Work out the finished part from the listing and answer in its coordinate system (mm). A direction names the side the tool comes from. Round coordinates to 2 decimals unless told otherwise and drop trailing zeros. Order: outer loops, then holes, each group sorted by start corner. A loop starts at its lowest first (then second) coordinate and runs counter-clockwise, first axis right, second up. Notation, with made-up numbers: M 21.25,-19 L 58.25,-19 A17 cw 58.25,-5 Z; hole C 33,-19 d2. An arc over 180 degrees is marked long. Return JSON: item names as keys, results as strings.
from build123d import *

# Parameters (mm, degrees)
BOX005_W                             = 145
BOX005_H                             = 15
BOX005_DEPTH                         = 182.3
BOX006_W                             = 19
BOX006_H                             = 163
BOX006_DEPTH                         = 13
BOX007_W                             = 112
BOX007_H                             = 172
BOX007_DEPTH                         = 1.5
BOX008_W                             = 11
BOX008_H                             = 32
BOX008_DEPTH                         = 2
BOX009_W                             = 3
BOX009_H                             = 24
BOX009_DEPTH                         = 17
BOX010_W                             = 60
BOX010_H                             = 32
BOX010_DEPTH                         = 5
BOX011_W                             = 15
BOX011_H                             = 80
BOX011_DEPTH                         = 5
BOX012_W                             = 5
BOX012_H                             = 70
BOX012_DEPTH                         = 3
LINEARPATTERN001_COUNT               = 2
LINEARPATTERN001_PITCH               = 80
FILLET_R                             = 1
FILLET001_R                          = 1
CYLINDER002_R                        = 1
CYLINDER002_DEPTH                    = 20
CYLINDER002_LINEARPATTERN002_2_R     = 1
CYLINDER002_LINEARPATTERN002_2_DEPTH = 20
LINEARPATTERN003_COUNT               = 2
LINEARPATTERN003_PITCH               = 170
BOX013_W                             = 11
BOX013_H                             = 165
BOX013_DEPTH                         = 4
CYLINDER004_R                        = 1
CYLINDER004_DEPTH                    = 3
CYLINDER004_LINEARPATTERN006_2_R     = 1
CYLINDER004_LINEARPATTERN006_2_DEPTH = 3
LINEARPATTERN007_COUNT               = 8
LINEARPATTERN007_PITCH               = 20
CYLINDER005_R                        = 3
CYLINDER005_DEPTH                    = 10
CYLINDER005_LINEARPATTERN008_2_R     = 3
CYLINDER005_LINEARPATTERN008_2_DEPTH = 10
LINEARPATTERN009_COUNT               = 2
LINEARPATTERN009_PITCH               = 170


with BuildPart() as part:
    # Box005 → Box005 (join)
    with BuildSketch(Plane(origin=(0, 182, -11), x_dir=(1, 0, 0), z_dir=(0, -1, 0))):
        with Locations((72.5, 7.5)):
            Rectangle(BOX005_W, BOX005_H)
    extrude(amount=BOX005_DEPTH)

    # Box006 → Box006 (cut)
    with BuildSketch(Plane(origin=(2, 8, -9), x_dir=(1, 0, 0), z_dir=(0, 0, 1))):
        with Locations((9.5, 81.5)):
            Rectangle(BOX006_W, BOX006_H)
    extrude(amount=BOX006_DEPTH, mode=Mode.SUBTRACT)

    # Box007 → Box007 (cut)
    with BuildSketch(Plane(origin=(23, 2, 2.5), x_dir=(1, 0, 0), z_dir=(0, 0, 1))):
        with Locations((56, 86)):
            Rectangle(BOX007_W, BOX007_H)
    extrude(amount=BOX007_DEPTH, mode=Mode.SUBTRACT)

    # Box008 → Box008 (cut)
    with BuildSketch(Plane(origin=(134, 69, 2), x_dir=(1, 0, 0), z_dir=(0, 0, 1))):
        with Locations((5.5, 16)):
            Rectangle(BOX008_W, BOX008_H)
    extrude(amount=BOX008_DEPTH, mode=Mode.SUBTRACT)

    # Box009 → Box009 (cut)
    with BuildSketch(Plane(origin=(142, 79, -12), x_dir=(1, 0, 0), z_dir=(0, 0, 1))):
        with Locations((1.5, 12)):
            Rectangle(BOX009_W, BOX009_H)
    extrude(amount=BOX009_DEPTH, mode=Mode.SUBTRACT)

    # Box010 → Box010 (cut)
    with BuildSketch(Plane(origin=(82, 75, -11), x_dir=(1, 0, 0), z_dir=(0, 0, 1))):
        with Locations((30, 16)):
            Rectangle(BOX010_W, BOX010_H)
    extrude(amount=BOX010_DEPTH, mode=Mode.SUBTRACT)

    # Box011 → Box011 (cut)
    with BuildSketch(Plane(origin=(82, -2, -11), x_dir=(1, 0, 0), z_dir=(0, 0, 1))):
        with Locations((7.5, 40)):
            Rectangle(BOX011_W, BOX011_H)
    extrude(amount=BOX011_DEPTH, mode=Mode.SUBTRACT)

    # Box012 → Box012 (cut)
    with BuildSketch(Plane(origin=(30, -1, -11), x_dir=(1, 0, 0), z_dir=(0, 0, 1))):
        with Locations((2.5, 35)):
            Rectangle(BOX012_W, BOX012_H)
    box012 = extrude(amount=BOX012_DEPTH, mode=Mode.SUBTRACT)

    # LinearPattern001: Box012 ×2
    with Locations(*[(i * LINEARPATTERN001_PITCH, 0, 0) for i in range(1, LINEARPATTERN001_COUNT)]):
        add(box012, mode=Mode.SUBTRACT)

    # Fillet
    fillet_edges = [part.edges().sort_by_distance(p)[0] for p in [
        (30, 34.35, -8),
        (32.5, 69, -8),
        (35, 34.35, -8),
        (32.5, -0.3, -8),
    ]]
    fillet(fillet_edges, radius=FILLET_R)

    # Fillet001
    fillet001_edges = [part.edges().sort_by_distance(p)[0] for p in [
        (110, 34.35, -8),
        (112.5, 69, -8),
        (115, 34.35, -8),
        (112.5, -0.3, -8),
    ]]
    fillet(fillet001_edges, radius=FILLET001_R)

    # Cylinder002 → Cylinder002 (cut)
    with BuildSketch(Plane(origin=(5, 5, -13), x_dir=(1, 0, 0), z_dir=(0, 0, 1))):
        Circle(CYLINDER002_R)
    cylinder002 = extrude(amount=CYLINDER002_DEPTH, mode=Mode.SUBTRACT)

    # Cylinder002 LinearPattern002 2 → Cylinder002 LinearPattern002 2 (cut)
    with BuildSketch(Plane(origin=(138, 5, -13), x_dir=(1, 0, 0), z_dir=(0, 0, 1))):
        Circle(CYLINDER002_LINEARPATTERN002_2_R)
    cylinder002_linearpattern002_2 = extrude(amount=CYLINDER002_LINEARPATTERN002_2_DEPTH, mode=Mode.SUBTRACT)

    # LinearPattern003: Cylinder002, Cylinder002 LinearPattern002 2 ×2
    with Locations(*[(0, i * LINEARPATTERN003_PITCH, 0) for i in range(1, LINEARPATTERN003_COUNT)]):
        add(cylinder002, mode=Mode.SUBTRACT)
        add(cylinder002_linearpattern002_2, mode=Mode.SUBTRACT)

    # Box013 → Box013 (join)
    with BuildSketch(Plane(origin=(4, 8, -9), x_dir=(1, 0, 0), z_dir=(0, 0, 1))):
        with Locations((5.5, 82.5)):
            Rectangle(BOX013_W, BOX013_H)
    extrude(amount=BOX013_DEPTH)

    # Cylinder004 → Cylinder004 (cut)
    with BuildSketch(Plane(origin=(9.125, 15.625, -8), x_dir=(1, 0, 0), z_dir=(0, 0, 1))):
        Circle(CYLINDER004_R)
    cylinder004 = extrude(amount=CYLINDER004_DEPTH, mode=Mode.SUBTRACT)

    # Cylinder004 LinearPattern006 2 → Cylinder004 LinearPattern006 2 (cut)
    with BuildSketch(Plane(origin=(9.125, 24.625, -8), x_dir=(1, 0, 0), z_dir=(0, 0, 1))):
        Circle(CYLINDER004_LINEARPATTERN006_2_R)
    cylinder004_linearpattern006_2 = extrude(amount=CYLINDER004_LINEARPATTERN006_2_DEPTH, mode=Mode.SUBTRACT)

    # LinearPattern007: Cylinder004, Cylinder004 LinearPattern006 2 ×8
    with Locations(*[(0, i * LINEARPATTERN007_PITCH, 0) for i in range(1, LINEARPATTERN007_COUNT)]):
        add(cylinder004, mode=Mode.SUBTRACT)
        add(cylinder004_linearpattern006_2, mode=Mode.SUBTRACT)

    # Cylinder005 → Cylinder005 (cut)
    with BuildSketch(Plane(origin=(5, 5, -12), x_dir=(1, 0, 0), z_dir=(0, 0, 1))):
        Circle(CYLINDER005_R)
    cylinder005 = extrude(amount=CYLINDER005_DEPTH, mode=Mode.SUBTRACT)

    # Cylinder005 LinearPattern008 2 → Cylinder005 LinearPattern008 2 (cut)
    with BuildSketch(Plane(origin=(138, 5, -12), x_dir=(1, 0, 0), z_dir=(0, 0, 1))):
        Circle(CYLINDER005_LINEARPATTERN008_2_R)
    cylinder005_linearpattern008_2 = extrude(amount=CYLINDER005_LINEARPATTERN008_2_DEPTH, mode=Mode.SUBTRACT)

    # LinearPattern009: Cylinder005, Cylinder005 LinearPattern008 2 ×2
    with Locations(*[(0, i * LINEARPATTERN009_PITCH, 0) for i in range(1, LINEARPATTERN009_COUNT)]):
        add(cylinder005, mode=Mode.SUBTRACT)
        add(cylinder005_linearpattern008_2, mode=Mode.SUBTRACT)


solid = part.part
Item 1: Consider line 1 along X through (y, z) = (5, 1.8); line 2 along X through (y, z) = (140.5, -7.5); line 3 along Y through (x, z) = (138, 0.95). Determine where each line is inside the solid, lowest interval first. Write a range as [from, to].
Output:
{"line 1": "x = [0, 4], [6, 137], [139, 145]", "line 2": "x = [0, 2], [4, 15], [21, 145]", "line 3": "y = [-0.3, 4], [6, 174], [176, 182]"}
Item 2: Find section B-B (y = 131.5). Determine the outline of the cut face in (x, z).
Output:
{"outline": "M 0,-11 L 145,-11 L 145,4 L 135,4 L 135,2.5 L 23,2.5 L 23,4 L 21,4 L 21,-9 L 15,-9 L 15,-5 L 4,-5 L 4,-9 L 2,-9 L 2,4 L 0,4 Z"}
Item 3: Find section A-A (x = 71). Determine the outline of the cut face in (y, z).
Output:
{"outline": "M -0.3,-11 L 182,-11 L 182,4 L 174,4 L 174,2.5 L 2,2.5 L 2,4 L -0.3,4 Z"}
Item 4: The mould has two halves that part along X. Classify faces 5 (the flat face through (82, 53, -9)), 6 (the flat face through (0, 92, -4)), 7 (the flat face through (71, 182, -3)): pulls with the +X half, pulls with the -X half, needs draft (parallel to the pull), parting line crosses it, or undercut.
Output:
{"face 5": "undercut", "face 6": "pulls with the -X half", "face 7": "needs draft"}
Item 5: Which of the six approach directions +Z, -Z, +X, -X, +Y, -Y give full straight-line access (tool end or side, diameter ignored) to faces 1 (the flat face through (78, 89, 2.5)), 2 (the flat face through (138, 85, 2)), 3 (the flat face through (145, 40, -4)), 4 (the flat face through (105, 78, -6))?
Output:
{"face 1": "+Z", "face 2": "+Z, +X", "face 3": "+Z, -Z, +X, +Y, -Y", "face 4": "-Z"}
Item 6: Each of these flat-tipped pins is pushed along its axis until it touches: pin 1 (6.5 mm diameter, centred on x = 4, y = 173.5, fed in from -Z); pin 2 (2 mm diameter, centred on x = 9.5, y = 164.5, fed in from +Z); pin 3 (0.6 mm diameter, centred on y = 91, z = 2, fed in from +X); pin 4 (0.6 mm diameter, centred on x = 32, z = -10.5, fed in from -Y). Where does it stop, or does it pass through?
Output:
{"pin 1": "stops at z = -11", "pin 2": "stops at z = -5", "pin 3": "stops at x = 142", "pin 4": "stops at y = 69"}
